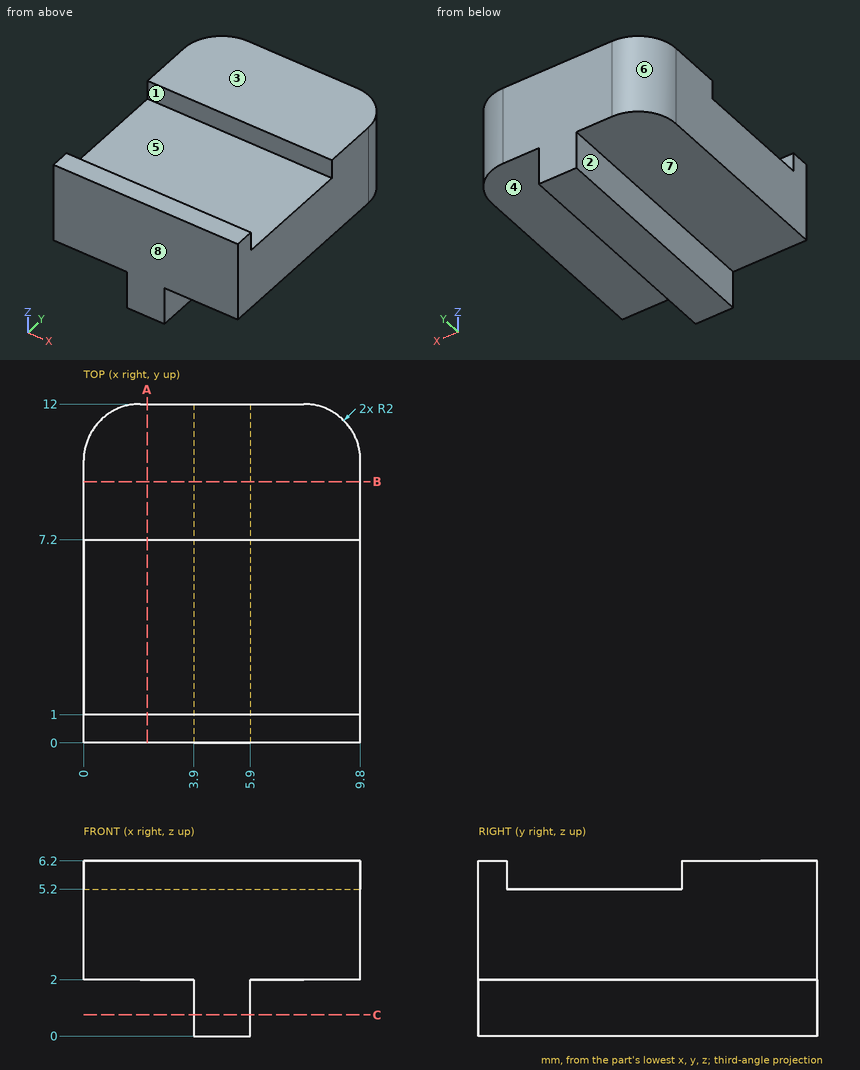
For this review, use the dimensioned drawing (mm, ordinates from the lowest corner) and the shaded views. A direction names the side the tool comes from. Coordinates: 2 decimals unless noted, no trailing zeros. Loops run counter-clockwise (first coordinate to the right, second up) from the corner with the lowest first, then second, coordinate; pieces in that order, holes last. Notation, with made-up numbers: M -39.5,43.5 L 0.5,43.5 A27 ccw 0.5,66.5 Z; hole C 12,71.25 d3. An arc over 180 degrees is marked long. Answer as CSV lines item,"result".
Item 1: The part is to be moulded in two halves that separate along Y. For the marked faces 5, 6, 7 and 8, say which applies: pulls with the +Y half, pulls with the -Y half, needs draft (parallel to the pull), parting line crosses it, or undercut.
Answer list:
face 5,"undercut"
face 6,"pulls with the +Y half"
face 7,"needs draft"
face 8,"pulls with the -Y half"
Item 2: Add section A-A on x = 2.25. State the section outline as (y, z) points, plus the area to 3 significant figures.
Answer list:
outline,"M 0,2 L 12,2 L 12,6.2 L 7.2,6.2 L 7.2,5.2 L 1,5.2 L 1,6.2 L 0,6.2 Z"
area,"44.2 mm²"
Item 3: For probe 1 along Y at (x, z) = (6.5, 5.75); probe 2 along X at (y, z) = (1, 1.75); probe 3 along Z at (x, y) = (5.5, 6.5), list the stretches that pass through material, from the lowest coordinate up.
Answer list:
probe 1,"0 to 1, 7.2 to 12"
probe 2,"3.9 to 5.9"
probe 3,"0 to 5.2"
Item 4: Add section B-B on y = 9.25. State the section outline as (x, z) points, plus the area to 3 significant figures.
Answer list:
outline,"M 0,2 L 3.9,2 L 3.9,0 L 5.9,0 L 5.9,2 L 9.8,2 L 9.8,6.2 L 0,6.2 Z"
area,"45.2 mm²"
Item 5: Add section C-C on z = 0.75. State the section outline as (x, y) points, plus the area to 3 significant figures.
Answer list:
outline,"M 3.9,0 L 5.9,0 L 5.9,12 L 3.9,12 Z"
area,"24.0 mm²"
Item 6: Machinability: for the marked faces 1, 2, 3 and 4, which of the approach directions +Z, -Z, +X, -X, +Y, -Y give a long, thin tool a straight path to every point of the face, cutting with its end or side? Answer none if there is none.
Answer list:
face 1,"+Z, +X, -X"
face 2,"-Z, -X, +Y, -Y"
face 3,"+Z, +X, -X, +Y, -Y"
face 4,"-Z, +X, +Y, -Y"
Item 7: For P1, Ø1.2, axis at x = 8, y = 4.5, coming from the -Z side; P2, Ø2, axis at y = 1.5, z = 0.5, coming from the -X side; P3, Ø1, axis at y = 9, z = 1, coming from the +X side, all flat-tipped, find the tip position at first contact; note any pin that passes through.
Answer list:
P1,"z = 2"
P2,"x = 3.9"
P3,"x = 5.9"
